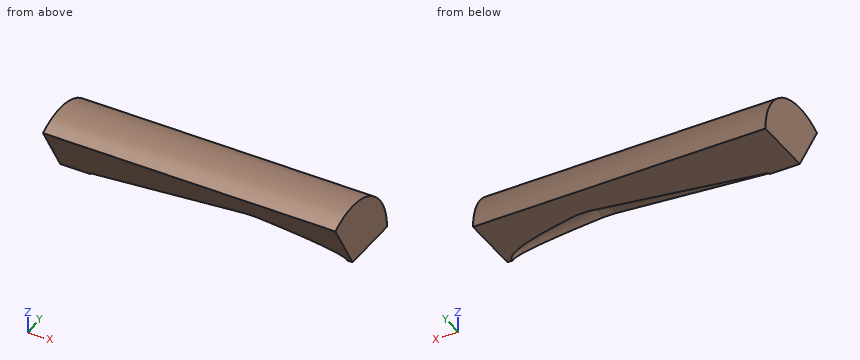
```python
from build123d import *

# Parameters (mm, degrees)
SKETCH1_W      = 44.45
SKETCH1_H      = 215.9
REVOLVE1_ANGLE = 120


with BuildPart() as part:
    # Sketch1 → Revolve1 (revolve)
    with BuildSketch(Plane(origin=(0, 0, 0), x_dir=(0, 1, 0), z_dir=(0, 0, 1))):
        with Locations((22.225, 107.95)):
            Rectangle(SKETCH1_W, SKETCH1_H)
    revolve(axis=Axis((0, 0, 0), (1, 0, 0)), revolution_arc=REVOLVE1_ANGLE)

    # Sketch21 → Cut-Revolve21 (revolve, cut)
    with BuildSketch(Plane(origin=(0, 0, 0), x_dir=(-1, 0, 0), z_dir=(0, 0, -1))):
        with BuildLine():
            Line((3.81, 0), (193.361475911, 0))
            Line((193.361475911, 0), (193.361555592, 1.489862296))
            Line((193.361555592, 1.489862296), (73.362678959, 22.496280175))
            Line((73.362678959, 22.496280175), (71.862679183, 22.500563741))
            Line((71.862679183, 22.500563741), (63.809813581, 22.500497032))
            add(Edge.make_bspline(
                [(3.81, 0), (3.409136339, 11.429131598), (63.809813581, 22.500497032)],
                knots=[0, 0, 0, 1, 1, 1], degree=2))
        make_face()
    revolve(axis=Axis((-215.9, 0, 0), (1, 0, 0)), mode=Mode.SUBTRACT)


solid = part.part
```
The listing builds one solid part. Answer for the finished solid, in the listing's coordinates (mm). Coordinates: 2 decimals unless noted, no trailing zeros. Order: outer loops, then holes, each group sorted by start corner. A loop starts at its lowest first (then second) coordinate and runs counter-clockwise, first axis right, second up. Notation, with made-up numbers: M -32.5,-28 L -24.5,-28 A16 ccw -24.5,-3 Z; hole C 42,2.25 d1. An arc over 180 degrees is marked long. Answer as a JSON object with one key per item and string values. Group by question number.
1. Straight lines are drawn through the part: line 1 (Z direction, x = -166.5, y = 6.5); line 2 (Y direction, x = -183.5, z = 12.5); line 3 (Y direction, x = -72, z = 23). For each, find the intervals that lie inside material, in ascending order.
2. Section B-B on z = 41.5 is taken. Write down the section's boundary in (x, y).
3. Flat-ended cylindrical pins translate along their axes: P1, Ø2, axis at x = -64, z = 9.5, coming from the +Y side; P2, Ø2, axis at x = -121, z = 34.5, coming from the -Y side; P3, Ø3, axis at x = -168, y = -14, coming from the +Z side. Find the tip coordinate at first contact, or state that the pin passes through.
4. Section A-A on x = -111 is taken. Write down the section's boundary in (y, z) (3 decimals).
Values follow:
{
 "1": {"line 1": "0 to 43.97", "line 2": "-7.22 to 42.66", "line 3": "-13.28 to 38.04"},
 "2": {"outline": "M -215.9,-15.92 L 0,-15.92 L 0,15.92 L -215.9,15.92 Z"},
 "3": {"P1": "y = 43.63", "P2": "y = -20.5", "P3": "z = 42.66"},
 "4": {"outline": "M -22.225,38.495 L -7.954,13.776 A15.908 cw 15.908,0 L 44.45,0 A44.45 ccw Z"}
}
